Autodesk Inventor part; units mm, degrees
ref_plane "YZ Plane" through (0, 0, 0) normal (1, 0, 0) x (0, 1, 0)
ref_plane "XZ Plane" through (0, 0, 0) normal (0, 1, 0) x (-1, 0, 0)
ref_plane "XY Plane" through (0, 0, 0) normal (0, 0, 1) x (1, 0, 0)
ref_plane "작업 평면1" through (0, 0, 0) normal (0, 0, 1) x (1, 0, 0)
sketch "스케치2" plane through (0, 0, 0) normal (0, 0, 1) x (1, 0, 0)
  line L0 (13.5, -39.75) -> (11.5, -39.75)
  arc A0 (11.5, -39.75) -> (9.25, -42) centre (11.5, -42) ccw
  line L1 (9.25, -42) -> (9.25, -44)
  arc A1 (8.25, -45) -> (9.25, -44) centre (8.25, -44) ccw
  line L2 (8.25, -45) -> (-8.25, -45)
  arc A2 (-9.25, -44) -> (-8.25, -45) centre (-8.25, -44) ccw
  line L3 (-9.25, -44) -> (-9.25, -42)
  arc A3 (-9.25, -42) -> (-11.5, -39.75) centre (-11.5, -42) ccw
  line L4 (-11.5, -39.75) -> (-13.5, -39.75)
  arc A4 (-14.5, -38.75) -> (-13.5, -39.75) centre (-13.5, -38.75) ccw
  line L5 (-14.5, -38.75) -> (-14.5, 8.25)
  arc A5 (-13.5, 9.25) -> (-14.5, 8.25) centre (-13.5, 8.25) ccw
  line L6 (-13.5, 9.25) -> (-11.5, 9.25)
  arc A6 (-11.5, 9.25) -> (-9.25, 11.5) centre (-11.5, 11.5) ccw
  line L7 (-9.25, 11.5) -> (-9.25, 14.5)
  line L8 (-15, 14.5) -> (-9.25, 14.5)
  line L9 (-20.1, 8.5) -> (-15, 14.5)
  line L10 (-20.1, -44.6) -> (-20.1, 8.5)
  line L11 (-15, -50.6) -> (-20.1, -44.6)
  line L12 (15, -50.6) -> (-15, -50.6)
  line L13 (20.1, -44.6) -> (15, -50.6)
  line L14 (20.1, 8.5) -> (20.1, -44.6)
  line L15 (15, 14.5) -> (20.1, 8.5)
  line L16 (9.25, 14.5) -> (15, 14.5)
  line L17 (9.25, 14.5) -> (9.25, 11.5)
  arc A7 (9.25, 11.5) -> (11.5, 9.25) centre (11.5, 11.5) ccw
  line L18 (11.5, 9.25) -> (13.5, 9.25)
  arc A8 (14.5, 8.25) -> (13.5, 9.25) centre (13.5, 8.25) ccw
  line L19 (14.5, 8.25) -> (14.5, -38.75)
  arc A9 (13.5, -39.75) -> (14.5, -38.75) centre (13.5, -38.75) ccw
  circle A10 centre (17.3, 4) radius 1.35
  circle A11 centre (17.3, -18) radius 1.35
  circle A12 centre (11, -47.8) radius 1.35
  circle A13 centre (-17.3, 4) radius 1.35
  circle A14 centre (-17.3, -18) radius 1.35
  circle A15 centre (-11, -47.8) radius 1.35
  circle A16 centre (17.3, -40) radius 1.35
  circle A17 centre (-17.3, -40) radius 1.35
  line L20 (-43, 2.0766) -> (-43, -42.1766)
  line L21 (-14.6, 8.25) -> (-14.6, -38.75)
  arc A18 (-14.6, -38.75) -> (-13.5, -39.85) centre (-13.5, -38.75) ccw
  line L22 (-13.5, -39.85) -> (-11.5, -39.85)
  arc A19 (-9.35, -42) -> (-11.5, -39.85) centre (-11.5, -42) ccw
  line L23 (-9.35, -42) -> (-9.35, -44)
  arc A20 (-9.35, -44) -> (-8.25, -45.1) centre (-8.25, -44) ccw
  line L24 (-8.25, -45.1) -> (8.25, -45.1)
  arc A21 (8.25, -45.1) -> (9.35, -44) centre (8.25, -44) ccw
  line L25 (9.35, -44) -> (9.35, -42)
  arc A22 (11.5, -39.85) -> (9.35, -42) centre (11.5, -42) ccw
  line L26 (11.5, -39.85) -> (13.5, -39.85)
  arc A23 (13.5, -39.85) -> (14.6, -38.75) centre (13.5, -38.75) ccw
  line L27 (14.6, -38.75) -> (14.6, 8.25)
  arc A24 (14.6, 8.25) -> (13.5, 9.35) centre (13.5, 8.25) ccw
  line L28 (13.5, 9.35) -> (11.5, 9.35)
  arc A25 (9.35, 11.5) -> (11.5, 9.35) centre (11.5, 11.5) ccw
  line L29 (9.35, 11.5) -> (9.35, 14.4)
  line L30 (9.35, 14.4) -> (14.9538, 14.4)
  line L31 (14.9538, 14.4) -> (20, 8.4632)
  line L32 (20, 8.4632) -> (20, -44.5632)
  line L33 (20, -44.5632) -> (14.9538, -50.5)
  line L34 (14.9538, -50.5) -> (-14.9538, -50.5)
  line L35 (-20, -15) -> (-20, 8.4632)
  line L36 (-20, 8.4632) -> (-14.9538, 14.4)
  line L37 (-14.9538, 14.4) -> (-9.35, 14.4)
  line L38 (-9.35, 14.4) -> (-9.35, 11.5)
  arc A26 (-11.5, 9.35) -> (-9.35, 11.5) centre (-11.5, 11.5) ccw
  line L39 (-11.5, 9.35) -> (-13.5, 9.35)
  arc A27 (-13.5, 9.35) -> (-14.6, 8.25) centre (-13.5, 8.25) ccw
  line L40 (-20, -15) -> (-14.6, -15)
  line L41 (-14.6, -15) -> (-14.6, -45)
  line L42 (-43, -15) -> (-20, -15)
  line L43 (-35, -45) -> (-35, -50.5)
  line L44 (-35, -50.5) -> (-14.6, -50.5)
  line L45 (-14.6, -50.5) -> (-14.6, -45)
  line L46 (-35, -45) -> (-35, -15)
  point P0 (0, 0)
  point P1 (-14.6, -38.75)
  point P2 (-14.6, -50.5)
  point P3 (-14.6, -38.75)
  dimension "d1" = 0.1
  dimension "d27" = 20.4
extrude "돌출8" add sketch "스케치2" along normal blind 3 contours L44 L43 L46 L42 L10 L11 | L11 L10 L42 L40 L21 L41 L45 L34 L44
sketch "스케치10" plane through (-35, -50.5, 0) normal (-1, 0, 0) x (0, 0, 1)
  arc A0 (-36.5808, 54.2636) -> (-37.1, 52.5766) centre (-34.1, 52.5766) ccw
  line L0 (-37.1, 8.3234) -> (-37.1, 52.5766)
  arc A1 (-37.1, 8.3234) -> (-36.5808, 6.6364) centre (-34.1, 8.3234) ccw
  line L1 (-32.8929, 1.2131) -> (-36.5808, 6.6364)
  arc A2 (-32.8929, 1.2131) -> (-30.4121, -0.1) centre (-30.4121, 2.9) ccw
  line L2 (-3.5879, -0.1) -> (-30.4121, -0.1)
  arc A3 (-3.5879, -0.1) -> (-1.1071, 1.2131) centre (-3.5879, 2.9) ccw
  line L3 (2.5808, 6.6364) -> (-1.1071, 1.2131)
  arc A4 (2.5808, 6.6364) -> (3.1, 8.3234) centre (0.1, 8.3234) ccw
  line L4 (3.1, 52.5766) -> (3.1, 8.3234)
  arc A5 (3.1, 52.5766) -> (2.5808, 54.2636) centre (0.1, 52.5766) ccw
  line L5 (-1.4047, 60.1246) -> (2.5808, 54.2636)
  arc A6 (-1.4047, 60.1246) -> (-3.0586, 61) centre (-3.0586, 59) ccw
  line L6 (-9.35, 61) -> (-3.0586, 61)
  arc A7 (-7.85, 59.5) -> (-9.35, 61) centre (-9.35, 59.5) ccw
  line L7 (-7.85, 59.5) -> (-7.85, 58)
  arc A8 (-7.85, 58) -> (-5.5, 55.65) centre (-5.5, 58) ccw
  line L8 (-5.5, 55.65) -> (-3.5, 55.65)
  arc A9 (-2.5, 54.65) -> (-3.5, 55.65) centre (-3.5, 54.65) ccw
  line L9 (-2.5, 54.65) -> (-2.5, 11.85)
  arc A10 (-3.5, 10.85) -> (-2.5, 11.85) centre (-3.5, 11.85) ccw
  line L10 (-3.5, 10.85) -> (-5.5, 10.85)
  arc A11 (-5.5, 10.85) -> (-7.85, 8.5) centre (-5.5, 8.5) ccw
  line L11 (-7.85, 8.5) -> (-7.85, 6.5)
  arc A12 (-8.85, 5.5) -> (-7.85, 6.5) centre (-8.85, 6.5) ccw
  line L12 (-8.85, 5.5) -> (-25.15, 5.5)
  arc A13 (-26.15, 6.5) -> (-25.15, 5.5) centre (-25.15, 6.5) ccw
  line L13 (-26.15, 6.5) -> (-26.15, 8.5)
  arc A14 (-26.15, 8.5) -> (-28.5, 10.85) centre (-28.5, 8.5) ccw
  line L14 (-28.5, 10.85) -> (-30.5, 10.85)
  arc A15 (-31.5, 11.85) -> (-30.5, 10.85) centre (-30.5, 11.85) ccw
  line L15 (-31.5, 11.85) -> (-31.5, 54.65)
  arc A16 (-30.5, 55.65) -> (-31.5, 54.65) centre (-30.5, 54.65) ccw
  line L16 (-30.5, 55.65) -> (-28.5, 55.65)
  arc A17 (-28.5, 55.65) -> (-26.15, 58) centre (-28.5, 58) ccw
  line L17 (-26.15, 58) -> (-26.15, 59.5)
  arc A18 (-24.65, 61) -> (-26.15, 59.5) centre (-24.65, 59.5) ccw
  line L18 (-30.9414, 61) -> (-24.65, 61)
  arc A19 (-30.9414, 61) -> (-32.5953, 60.1246) centre (-30.9414, 59) ccw
  line L19 (-36.5808, 54.2636) -> (-32.5953, 60.1246)
  circle A20 centre (0.3, 52) radius 1.35
  circle A21 centre (0.3, 30) radius 1.35
  circle A22 centre (-6, 2.7) radius 1.35
  circle A23 centre (-34.3, 52) radius 1.35
  circle A24 centre (-34.3, 30) radius 1.35
  circle A25 centre (-28, 2.7) radius 1.35
  circle A26 centre (0.3, 8) radius 1.35
  circle A27 centre (-34.3, 8) radius 1.35
  line L20 (0, 35.5) -> (0, 0)
  line L21 (0, 0) -> (3, 0)
  line L22 (3, 35.5) -> (3, 0)
  line L23 (0, 35.5) -> (3, 35.5)
  line L24 (-2.4, 11.85) -> (-2.4, 54.65)
  arc A28 (-2.4, 54.65) -> (-3.5, 55.75) centre (-3.5, 54.65) ccw
  line L25 (-3.5, 55.75) -> (-5.5, 55.75)
  arc A29 (-7.75, 58) -> (-5.5, 55.75) centre (-5.5, 58) ccw
  line L26 (-7.75, 58) -> (-7.75, 59.5)
  arc A30 (-7.75, 59.5) -> (-10.1246, 60.9) centre (-9.35, 59.5) ccw
  line L27 (-10.1246, 60.9) -> (-3.0586, 60.9)
  arc A31 (-1.4874, 60.0684) -> (-3.0586, 60.9) centre (-3.0586, 59) ccw
  line L28 (-1.4874, 60.0684) -> (2.4981, 54.2073)
  arc A32 (3, 52.5766) -> (2.4981, 54.2073) centre (0.1, 52.5766) ccw
  line L29 (3, 52.5766) -> (3, 8.3234)
  arc A33 (2.4981, 6.6927) -> (3, 8.3234) centre (0.1, 8.3234) ccw
  line L30 (2.4981, 6.6927) -> (0, 3.019)
  arc A34 (-3.5879, 0) -> (-2.4, 0.2545) centre (-3.5879, 2.9) ccw
  line L31 (-3.5879, 0) -> (-30.4121, 0)
  arc A35 (-32.8102, 1.2693) -> (-30.4121, 0) centre (-30.4121, 2.9) ccw
  line L32 (-32.8102, 1.2693) -> (-36.4981, 6.6927)
  arc A36 (-37, 8.3234) -> (-36.4981, 6.6927) centre (-34.1, 8.3234) ccw
  line L33 (-37, 8.3234) -> (-37, 52.5766)
  arc A37 (-36.4981, 54.2073) -> (-37, 52.5766) centre (-34.1, 52.5766) ccw
  line L34 (-36.4981, 54.2073) -> (-32.5126, 60.0684)
  arc A38 (-30.9414, 60.9) -> (-32.5126, 60.0684) centre (-30.9414, 59) ccw
  line L35 (-30.9414, 60.9) -> (-25.4246, 60.9)
  arc A39 (-25.4246, 60.9) -> (-26.25, 59.5) centre (-24.65, 59.5) ccw
  line L36 (-26.25, 59.5) -> (-26.25, 58)
  arc A40 (-28.5, 55.75) -> (-26.25, 58) centre (-28.5, 58) ccw
  line L37 (-28.5, 55.75) -> (-30.5, 55.75)
  arc A41 (-30.5, 55.75) -> (-31.6, 54.65) centre (-30.5, 54.65) ccw
  line L38 (-31.6, 54.65) -> (-31.6, 11.85)
  arc A42 (-31.6, 11.85) -> (-30.5, 10.75) centre (-30.5, 11.85) ccw
  line L39 (-30.5, 10.75) -> (-28.5, 10.75)
  arc A43 (-26.25, 8.5) -> (-28.5, 10.75) centre (-28.5, 8.5) ccw
  line L40 (-26.25, 8.5) -> (-26.25, 6.5)
  arc A44 (-26.25, 6.5) -> (-25.15, 5.4) centre (-25.15, 6.5) ccw
  line L41 (-25.15, 5.4) -> (-8.85, 5.4)
  arc A45 (-8.85, 5.4) -> (-7.75, 6.5) centre (-8.85, 6.5) ccw
  line L42 (-7.75, 6.5) -> (-7.75, 8.5)
  arc A46 (-5.5, 10.75) -> (-7.75, 8.5) centre (-5.5, 8.5) ccw
  line L43 (-5.5, 10.75) -> (-3.5, 10.75)
  arc A47 (-3.5, 10.75) -> (-2.4, 11.85) centre (-3.5, 11.85) ccw
  line L44 (0, 0) -> (-2.4, 0)
  line L45 (-2.4, 0) -> (-2.4, 35.5)
  line L46 (-2.4, 35.5) -> (0, 35.5)
  line L47 (0, 35.5) -> (0, 0)
  point P0 (0, 50.5)
  point P1 (0, 6.6838)
  point P2 (0, 9.3162)
  point P3 (0, 28.6838)
  point P4 (0, 31.3162)
  point P5 (0, 35.5)
  point P6 (-2.4, 11.85)
  dimension "d30" = 0.1
extrude "돌출10" add sketch "스케치10" against normal blind 12 contours L45 L24 L46 L20 A21 A26 L3 A3 | A3 L3 L20 L44 L45
sketch "스케치12" plane through (-35, -50.5, 3) normal (-1, 0, 0) x (0, 0, 1)
  line L0 (-5.5579, 8) -> (-4.1289, 5.525)
  arc A0 (-39.5808, 54.2636) -> (-40.1, 52.5766) centre (-37.1, 52.5766) ccw
  line L1 (-40.1, 8.3234) -> (-40.1, 52.5766)
  arc A1 (-40.1, 8.3234) -> (-39.5808, 6.6364) centre (-37.1, 8.3234) ccw
  line L2 (-35.8929, 1.2131) -> (-39.5808, 6.6364)
  arc A2 (-35.8929, 1.2131) -> (-33.4121, -0.1) centre (-33.4121, 2.9) ccw
  line L3 (-6.5879, -0.1) -> (-33.4121, -0.1)
  arc A3 (-6.5879, -0.1) -> (-4.1071, 1.2131) centre (-6.5879, 2.9) ccw
  line L4 (-0.4192, 6.6364) -> (-4.1071, 1.2131)
  arc A4 (-0.4192, 6.6364) -> (0.1, 8.3234) centre (-2.9, 8.3234) ccw
  line L5 (0.1, 52.5766) -> (0.1, 8.3234)
  arc A5 (0.1, 52.5766) -> (-0.4192, 54.2636) centre (-2.9, 52.5766) ccw
  line L6 (-4.4047, 60.1246) -> (-0.4192, 54.2636)
  arc A6 (-4.4047, 60.1246) -> (-6.0586, 61) centre (-6.0586, 59) ccw
  line L7 (-12.35, 61) -> (-6.0586, 61)
  arc A7 (-10.85, 59.5) -> (-12.35, 61) centre (-12.35, 59.5) ccw
  line L8 (-10.85, 59.5) -> (-10.85, 58)
  arc A8 (-10.85, 58) -> (-8.5, 55.65) centre (-8.5, 58) ccw
  line L9 (-8.5, 55.65) -> (-6.5, 55.65)
  arc A9 (-5.5, 54.65) -> (-6.5, 55.65) centre (-6.5, 54.65) ccw
  line L10 (-5.5, 54.65) -> (-5.5, 11.85)
  arc A10 (-6.5, 10.85) -> (-5.5, 11.85) centre (-6.5, 11.85) ccw
  line L11 (-6.5, 10.85) -> (-8.5, 10.85)
  arc A11 (-8.5, 10.85) -> (-10.85, 8.5) centre (-8.5, 8.5) ccw
  line L12 (-10.85, 8.5) -> (-10.85, 6.5)
  arc A12 (-11.85, 5.5) -> (-10.85, 6.5) centre (-11.85, 6.5) ccw
  line L13 (-11.85, 5.5) -> (-28.15, 5.5)
  arc A13 (-29.15, 6.5) -> (-28.15, 5.5) centre (-28.15, 6.5) ccw
  line L14 (-29.15, 6.5) -> (-29.15, 8.5)
  arc A14 (-29.15, 8.5) -> (-31.5, 10.85) centre (-31.5, 8.5) ccw
  line L15 (-31.5, 10.85) -> (-33.5, 10.85)
  arc A15 (-34.5, 11.85) -> (-33.5, 10.85) centre (-33.5, 11.85) ccw
  line L16 (-34.5, 11.85) -> (-34.5, 54.65)
  arc A16 (-33.5, 55.65) -> (-34.5, 54.65) centre (-33.5, 54.65) ccw
  line L17 (-33.5, 55.65) -> (-31.5, 55.65)
  arc A17 (-31.5, 55.65) -> (-29.15, 58) centre (-31.5, 58) ccw
  line L18 (-29.15, 58) -> (-29.15, 59.5)
  arc A18 (-27.65, 61) -> (-29.15, 59.5) centre (-27.65, 59.5) ccw
  line L19 (-33.9414, 61) -> (-27.65, 61)
  arc A19 (-33.9414, 61) -> (-35.5953, 60.1246) centre (-33.9414, 59) ccw
  line L20 (-39.5808, 54.2636) -> (-35.5953, 60.1246)
  circle A20 centre (-2.7, 52) radius 1.35
  circle A21 centre (-2.7, 30) radius 1.35
  circle A22 centre (-9, 2.7) radius 1.35
  circle A23 centre (-37.3, 52) radius 1.35
  circle A24 centre (-37.3, 30) radius 1.35
  circle A25 centre (-31, 2.7) radius 1.35
  circle A26 centre (-2.7, 8) radius 1.35
  circle A27 centre (-37.3, 8) radius 1.35
  circle A28 centre (-2.7, 8) radius 1.35
  circle A29 centre (-2.7, 30) radius 1.35
  point P0 (-3, 50.5)
  dimension "d35" = 2.7
  dimension "d36" = 2.7
extrude "돌출11" cut sketch "스케치12" against normal blind 10 contours A21 | A26
sketch "스케치13" plane through (0, 0, 3) normal (0, 0, 1) x (1, 0, 0)
  line L0 (-25, -43.85) -> (-35, -43.85)
  line L1 (-25, -41.15) -> (-35, -41.15)
  line L2 (-25, -21.85) -> (-35, -21.85)
  line L3 (-25, -19.15) -> (-35, -19.15)
  line L4 (-30, -43.85) -> (-30, -41.15)
  line L5 (-30, -19.15) -> (-30, -21.85)
  line L6 (-28.9, -39.9) -> (-31.1, -39.9)
  line L7 (-31.1, -39.9) -> (-31.1, -45.1)
  line L8 (-31.1, -45.1) -> (-28.9, -45.1)
  line L9 (-28.9, -45.1) -> (-28.9, -39.9)
  line L10 (-28.9, -39.9) -> (-31.1, -45.1) construction
  line L11 (-31.1, -39.9) -> (-28.9, -45.1) construction
  line L12 (-28.9, -17.9) -> (-31.1, -17.9)
  line L13 (-31.1, -17.9) -> (-31.1, -23.1)
  line L14 (-31.1, -23.1) -> (-28.9, -23.1)
  line L15 (-28.9, -23.1) -> (-28.9, -17.9)
  line L16 (-28.9, -17.9) -> (-31.1, -23.1) construction
  line L17 (-31.1, -17.9) -> (-28.9, -23.1) construction
  point P0 (0, 0)
  point P1 (-30, -42.5)
  point P2 (-30, -20.5)
  dimension "d39" = 2.2
  dimension "d40" = 5.2
  dimension "d41" = 2.2
  dimension "d42" = 5.2
extrude "돌출12" cut sketch "스케치13" against normal blind 10
properties part number "foot_right_connection" material "PMMA 플라스틱"
Work out the finished part from the listing and answer in its coordinate system (mm). A direction names the side the tool comes from. Give positions to 0.01 mm unless a question says otherwise; leave off trailing zeros. Write each loop counter-clockwise with the first axis right and the second up, starting at its lowest first coordinate (ties: lowest second). Pieces come first, ordered by that corner, then holes.
(1) Flat-ended cylindrical pins translate along their axes: pin 1 Ø0.8 at (y, z) = (-20.5, 0.5) entering from -X; pin 2 Ø2 at (x, y) = (-20.5, -38.5) entering from -Z; pin 3 Ø5 at (x, y) = (-30, -22) entering from +Z; pin 4 Ø2 at (x, y) = (-17.3, -18) entering from +Z. Find the tip coordinate at first contact, or state that the pin passes through.
Final values:
pin 1: stops at x = -25
pin 2: stops at z = 0
pin 3: stops at z = 3
pin 4: passes through
(2) The part is cut by section B-B on z = 2.15. Write down the section's boundary in (x, y).
Final values:
outline: (-35, -50.5) - (-14.6, -50.5) - (-14.6, -15) - (-35, -15) - close; hole (-31.1, -45.1) - (-28.9, -45.1) - (-28.9, -39.9) - (-31.1, -39.9) - close; hole (-31.1, -23.1) - (-28.9, -23.1) - (-28.9, -17.9) - (-31.1, -17.9) - close; hole circle Ø2.7 at (-17.3, -40); hole circle Ø2.7 at (-17.3, -18)
(3) The part is cut by section D-D on z = -1.9. Write down the section's boundary in (x, y), plus the area to 3 significant figures.
Final values:
outline: (-35, -50.5) - (-23, -50.5) - (-23, -15) - (-35, -15) - close; hole (-31.1, -45.1) - (-28.9, -45.1) - (-28.9, -39.9) - (-31.1, -39.9) - close; hole (-31.1, -23.1) - (-28.9, -23.1) - (-28.9, -17.9) - (-31.1, -17.9) - close
area: 403 mm2
(4) The part is cut by section C-C on x = -32.75. Write down the section's boundary in (y, z).
Final values:
outline: (-50.5, -2.4) - (-15, -2.4) - (-15, 3) - (-50.5, 3) - close; hole circle Ø2.7 at (-42.5, 0.3); hole circle Ø2.7 at (-20.5, 0.3)
(5) The mould has two halves that part along Y. Classify faces 4 (the flat face through (-23, -33, -1)), 5 (the flat face through (-28.9, -22, 1)), 6 (the flat face through (-27, -50.5, 1)): pulls with the +Y half, pulls with the -Y half, needs draft (parallel to the pull), parting line crosses it, or undercut.
Final values:
face 4: needs draft
face 5: undercut
face 6: pulls with the -Y half
(6) Which of the six approach directions +Z, -Z, +X, -X, +Y, -Y give full straight-line access (tool end or side, diameter ignored) to faces 1 (the flat face through (-31.1, -41, 1)), 2 (the flat face through (-14.6, -33, 1)), 3 (the flat face through (-25, -20, 1))?
Final values:
face 1: +Z, -Z
face 2: +Z, -Z, +X, +Y, -Y
face 3: -X
(7) Straight lines are drawn through the part: line 1 (Y direction, x = -17.3, z = 2.15); line 2 (Y direction, x = -33.85, z = 0.3); line 3 (X direction, y = -22, z = -1.45). For each, find the intervals that lie inside material, in ascending order.
Final values:
line 1: y = -50.5 to -41.35, -38.65 to -19.35, -16.65 to -15
line 2: y = -50.5 to -43.85, -41.15 to -21.85, -19.15 to -15
line 3: x = -35 to -31.1, -28.9 to -23
(8) The part is cut by section A-A on y = -20.5. Write down the section's boundary in (x, z).
Final values:
outline: (-35, -2.4) - (-31.1, -2.4) - (-31.1, -1.05) - (-35, -1.05) - close; (-35, 1.65) - (-31.1, 1.65) - (-31.1, 3) - (-35, 3) - close; (-28.9, -2.4) - (-23, -2.4) - (-23, -1.05) - (-28.9, -1.05) - close; (-28.9, 1.65) - (-25, 1.65) - (-25, 0) - (-14.6, 0) - (-14.6, 3) - (-28.9, 3) - close
